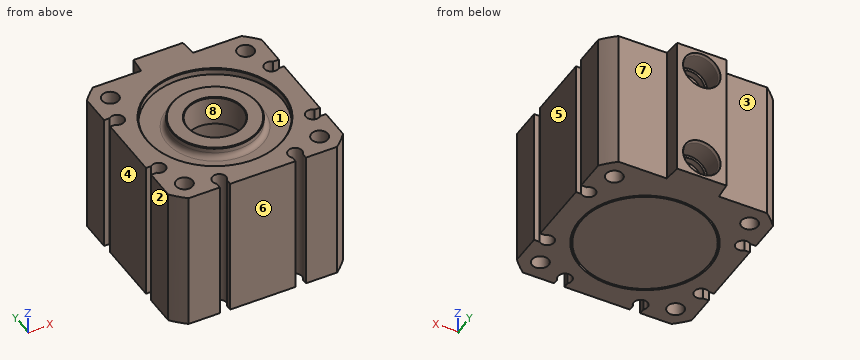
from build123d import *

# Parameters (mm, degrees)
EXTRUDE1_DEPTH                               = 20.701
EXTRUDE1_DEPTH_BACK                          = 20.701
SKETCH1_W                                    = 50.8
SKETCH1_H                                    = 50.8
F_056_250_NOSE_CHAMFER_R                     = 1.5
SKETCH13_R                                   = 35.921024484
SKETCH13_R_2                                 = 33.34
F_075_250_TUBE_EDGE_ROUNDOVER_DEPTH          = 55.812823354
F_075_250_PORT_BOSS_DEPTH                    = 41.402
F_106_200_PORT_1_8_NPT_AT_2_COUNT            = 2
F_106_200_PORT_1_8_NPT_AT_2_PITCH            = 28.702
F_075_250_SWITCH_GROOVE_DEPTH                = 58.174392905
F_075_106_SWITCH_GROOVE_CIRC_PATTERN_COUNT   = 3
F_075_106_SWITCH_GROOVE_CIRC_PATTERN_ANGLE   = 180
SKETCH19_W                                   = 0.15
SKETCH19_H                                   = 19
F_075_250_THIN_SIDE_CUTS_DEPTH               = 58.174392905
SKETCH20_R                                   = 1.9
F_075_250_MOUNT_THRU_HOLE_DEPTH              = 58.174392905
F_075_250_MOUNT_THRU_HOLE_CIRC_PATTERN_COUNT = 4
F_150_10_24_A_MOUNT_TAPPED_AT_2_COUNT        = 2
F_150_10_24_A_MOUNT_TAPPED_AT_2_PITCH        = 39.29
F_150_10_24_A_MOUNT_TAPPED_AT_3_COUNT        = 2
F_150_10_24_A_MOUNT_TAPPED_AT_3_PITCH        = 55.564450866
F_150_10_24_A_MOUNT_TAPPED_AT_4_COUNT        = 2
F_150_10_24_A_MOUNT_TAPPED_AT_4_PITCH        = 39.29
F_056_250_START                              = -12.025
SKETCH22_R                                   = 19.05
F_056_250_STROKE_CHAMBER_DEPTH               = 24.05
SKETCH23_R                                   = 8.001
F_056_250_ROD_THRU_BORE_DEPTH                = 45.534447353
SKETCH41_R                                   = 19.05
SKETCH41_R_2                                 = 18.55
END_PLATE_DEPTH                              = 1
END_PLATE_TAPER                              = 30
F_056_250_COLLAR_CHAMFER_SIZE                = 0.2


with BuildPart() as part:
    # Sketch1 → Extrude1 (new, two sides: drawn at the far end of the back side and taken through both)
    with BuildSketch(Plane.XY.offset(-EXTRUDE1_DEPTH_BACK)):
        Rectangle(SKETCH1_W, SKETCH1_H)
    extrude(amount=EXTRUDE1_DEPTH + EXTRUDE1_DEPTH_BACK)

    # Sketch33 → 056-250 Front Recess (revolve, cut)
    with BuildSketch(Plane(origin=(0, 0, 0), x_dir=(0, 0, -1), z_dir=(1, 0, 0)), mode=Mode.PRIVATE) as f_056_250_front_recess_sk:
        Polygon((-20.701, 19.55), (-18.801, 19.55), (-18.801, 21), (-17.651, 21), (-17.651, 12.5), (-20.701, 12.5), align=None)
    revolve(f_056_250_front_recess_sk.sketch.rotate(Axis((0, 0, 61.220394237), (0, 0, -1)), 90), axis=Axis((0, 0, 61.220394237), (0, 0, -1)), mode=Mode.SUBTRACT)

    # 056-250 Nose Chamfer
    f_056_250_nose_chamfer_edges = [part.edges().sort_by_distance(p)[0] for p in [
        (-12.5, 0, 17.651),
    ]]
    fillet(f_056_250_nose_chamfer_edges, radius=F_056_250_NOSE_CHAMFER_R)

    # Sketch13 → 075-250 Tube Edge Roundover (cut, through all)
    with BuildSketch(Plane.XY.offset(20.701)):
        Circle(SKETCH13_R)
        Circle(SKETCH13_R_2, mode=Mode.SUBTRACT)
    extrude(amount=-F_075_250_TUBE_EDGE_ROUNDOVER_DEPTH, mode=Mode.SUBTRACT)

    # Sketch14 → 075-250 Port Boss (add)
    with BuildSketch(Plane.XY.offset(20.701)):
        Polygon((-7.15, 30.16), (7.15, 30.16), (7.566446038, 25.4), (-7.566446038, 25.4), align=None)
    extrude(amount=-F_075_250_PORT_BOSS_DEPTH)

    # Sketch36 → 106-200 Port 1/8 NPT (revolve, cut)
    with BuildSketch(Plane(origin=(0, 30.16, 14.351), x_dir=(0, 0, 1), z_dir=(1, 0, 0))):
        Polygon((0, 0), (0, 10.533468714), (4.2164, 8), (4.2164, 6.2), (4.959907269, 6.2), (5.1218211, 0.792298297), (5.4500018, 0), align=None)
    f_106_200_port_1_8_npt = revolve(axis=Axis((0, 36.51, 14.351), (0, -1, 0)), mode=Mode.SUBTRACT)

    # 106-200 Port 1/8 NPT at 2: 106-200 Port 1/8 NPT ×2
    with Locations(*[(0, 0, -i * F_106_200_PORT_1_8_NPT_AT_2_PITCH) for i in range(1, F_106_200_PORT_1_8_NPT_AT_2_COUNT)]):
        add(f_106_200_port_1_8_npt, mode=Mode.SUBTRACT)

    # Sketch15 → 075-250 Switch Groove (cut, through all)
    with BuildSketch(Plane.XY.offset(20.701)):
        with BuildLine():
            Line((-25.4, 12.5), (-23.760376786, 12.5))
            ThreePointArc((-23.760376786, 12.5), (-20.375, 11), (-23.760376786, 9.5))
            Line((-23.760376786, 9.5), (-25.4, 9.5))
            Line((-25.4, 9.5), (-25.4, 12.5))
        make_face()
        with BuildLine():
            Line((-25.4, -12.5), (-25.4, -9.5))
            Line((-25.4, -9.5), (-23.760376786, -9.5))
            ThreePointArc((-23.760376786, -9.5), (-20.375, -11), (-23.760376786, -12.5))
            Line((-23.760376786, -12.5), (-25.4, -12.5))
        make_face()
    f_075_250_switch_groove = extrude(amount=-F_075_250_SWITCH_GROOVE_DEPTH, mode=Mode.SUBTRACT)

    # 075-106 Switch Groove Circ Pattern: 075-250 Switch Groove ×3 about axis
    f_075_106_switch_groove_circ_pattern_axis = Axis((0, 0, 0), (0, 0, 1))
    for i in range(1, F_075_106_SWITCH_GROOVE_CIRC_PATTERN_COUNT):
        add(f_075_250_switch_groove.rotate(f_075_106_switch_groove_circ_pattern_axis, i * F_075_106_SWITCH_GROOVE_CIRC_PATTERN_ANGLE / (F_075_106_SWITCH_GROOVE_CIRC_PATTERN_COUNT - 1)), mode=Mode.SUBTRACT)

    # Sketch19 → 075-250 Thin Side Cuts (cut, through all)
    with BuildSketch(Plane.XY.offset(20.701)):
        with Locations((25.325, 0)):
            Rectangle(SKETCH19_W, SKETCH19_H)
        with Locations((-25.325, 0)):
            Rectangle(SKETCH19_W, SKETCH19_H)
    extrude(amount=-F_075_250_THIN_SIDE_CUTS_DEPTH, mode=Mode.SUBTRACT)

    # Sketch20 → 075-250 Mount Thru Hole (cut, through all)
    with BuildSketch(Plane.XY.offset(20.701)):
        with Locations((19.645, 19.645)):
            Circle(SKETCH20_R)
    f_075_250_mount_thru_hole = extrude(amount=-F_075_250_MOUNT_THRU_HOLE_DEPTH, mode=Mode.SUBTRACT)

    # 075-250 Mount Thru Hole Circ Pattern: 075-250 Mount Thru Hole ×4 about axis
    f_075_250_mount_thru_hole_circ_pattern_axis = Axis((0, 0, 0), (0, 0, 1))
    for i in range(1, F_075_250_MOUNT_THRU_HOLE_CIRC_PATTERN_COUNT):
        add(f_075_250_mount_thru_hole.rotate(f_075_250_mount_thru_hole_circ_pattern_axis, i * 360 / F_075_250_MOUNT_THRU_HOLE_CIRC_PATTERN_COUNT), mode=Mode.SUBTRACT)

    # Sketch28 → 150 #10-24 A Mount Tapped (revolve, cut)
    with BuildSketch(Plane(origin=(19.645, 19.645, 20.701), x_dir=(0, -1, 0), z_dir=(1, 0, 0))):
        Polygon((0, 0), (0, 17.018324014), (1.89865, 15.8775), (1.89865, 12.7), (2.413, 12.7), (2.413, 0), align=None)
    f_150_10_24_a_mount_tapped = revolve(axis=Axis((19.645, 19.645, 27.051), (0, 0, -1)), mode=Mode.SUBTRACT)

    # 150 #10-24 A Mount Tapped at 2: 150 #10-24 A Mount Tapped ×2
    with Locations(*[(-i * F_150_10_24_A_MOUNT_TAPPED_AT_2_PITCH, 0, 0) for i in range(1, F_150_10_24_A_MOUNT_TAPPED_AT_2_COUNT)]):
        add(f_150_10_24_a_mount_tapped, mode=Mode.SUBTRACT)

    # 150 #10-24 A Mount Tapped at 3: 150 #10-24 A Mount Tapped ×2
    with Locations(*[Vector(-0.7071067811865451, -0.7071067811865499, 0) * (i * F_150_10_24_A_MOUNT_TAPPED_AT_3_PITCH) for i in range(1, F_150_10_24_A_MOUNT_TAPPED_AT_3_COUNT)]):
        add(f_150_10_24_a_mount_tapped, mode=Mode.SUBTRACT)

    # 150 #10-24 A Mount Tapped at 4: 150 #10-24 A Mount Tapped ×2
    with Locations(*[(0, -i * F_150_10_24_A_MOUNT_TAPPED_AT_4_PITCH, 0) for i in range(1, F_150_10_24_A_MOUNT_TAPPED_AT_4_COUNT)]):
        add(f_150_10_24_a_mount_tapped, mode=Mode.SUBTRACT)

    # 150 #10-24 A Mount Tapped to Rear: 150 #10-24 A Mount Tapped across plane
    add(f_150_10_24_a_mount_tapped.mirror(Plane.XY), mode=Mode.SUBTRACT)

    # 150 #10-24 A Mount Tapped to Rear copy 1 → 150 #10-24 A Mount Tapped to Rear co 2 (revolve, cut)
    with BuildSketch(Plane(origin=(-19.645, 19.645, -20.701), x_dir=(0, -1, 0), z_dir=(1, 0, 0))):
        Polygon((0, 0), (0, -17.018324014), (1.89865, -15.8775), (1.89865, -12.7), (2.413, -12.7), (2.413, 0), align=None)
    revolve(axis=Axis((-19.645, 19.645, -27.051), (0, 0, -1)), mode=Mode.SUBTRACT)

    # 150 #10-24 A Mount Tapped to Rear copy 2 → 150 #10-24 A Mount Tapped to Rear co 3 (revolve, cut)
    with BuildSketch(Plane(origin=(-19.645, -19.645, -20.701), x_dir=(0, -1, 0), z_dir=(1, 0, 0))):
        Polygon((0, 0), (0, -17.018324014), (1.89865, -15.8775), (1.89865, -12.7), (2.413, -12.7), (2.413, 0), align=None)
    revolve(axis=Axis((-19.645, -19.645, -27.051), (0, 0, -1)), mode=Mode.SUBTRACT)

    # 150 #10-24 A Mount Tapped to Rear copy 3 → 150 #10-24 A Mount Tapped to Rear co 4 (revolve, cut)
    with BuildSketch(Plane(origin=(19.645, -19.645, -20.701), x_dir=(0, -1, 0), z_dir=(1, 0, 0))):
        Polygon((0, 0), (0, -17.018324014), (1.89865, -15.8775), (1.89865, -12.7), (2.413, -12.7), (2.413, 0), align=None)
    revolve(axis=Axis((19.645, -19.645, -27.051), (0, 0, -1)), mode=Mode.SUBTRACT)

    # Sketch22 → 056-250 Stroke Chamber (cut)
    with BuildSketch(Plane.XY.offset(F_056_250_START)):
        Circle(SKETCH22_R)
    extrude(amount=F_056_250_STROKE_CHAMBER_DEPTH, mode=Mode.SUBTRACT)

    # Sketch23 → 056-250 Rod Thru Bore (cut, through all)
    with BuildSketch(Plane.XY):
        Circle(SKETCH23_R)
    extrude(amount=F_056_250_ROD_THRU_BORE_DEPTH, mode=Mode.SUBTRACT)

    # Sketch41 → End Plate (cut)
    with BuildSketch(Plane(origin=(0, 0, -20.701), x_dir=(-1, 0, 0), z_dir=(0, 0, -1))):
        with Locations(Location((0, 0, 0), (0, 0, 180))):
            Circle(SKETCH41_R)
        Circle(SKETCH41_R_2, mode=Mode.SUBTRACT)
    extrude(amount=-END_PLATE_DEPTH, taper=END_PLATE_TAPER, mode=Mode.SUBTRACT)

    # 056-250 Collar Chamfer
    f_056_250_collar_chamfer_edges = [part.edges().sort_by_distance(p)[0] for p in [
        (-19.55, 0, 20.701),
        (-12.5, 0, 20.701),
        (-8.001, 0, 20.701),
    ]]
    chamfer(f_056_250_collar_chamfer_edges, length=F_056_250_COLLAR_CHAMFER_SIZE)


solid = part.part
Here's how the part is built. I have some questions about the finished solid (model axes, mm). Face numbers are marked on the shaded views. A direction names the side the tool comes from. Round coordinates to 2 decimals unless told otherwise and drop trailing zeros.
1. Suppose I cut it at A-A (z = -1.5). State how many separate pieces and enclosed holes the cut face has, and give its area (3 significant figures).
2. Will these pins go through, and if not, where does the flat tip stop? pin 1 Ø1.8 at (x, z) = (-24.5, -8) entering from +Y; pin 2 Ø1.8 at (x, z) = (-24.5, -3.5) entering from -Y; pin 3 Ø15 at (y, z) = (-0.5, 5.5) entering from -X.
3. I need wall thicknesses on L1, parallel to X at y = -19.5, z = 10; L2, parallel to X at y = 20, z = -6.5; L3, parallel to Y at x = 22.5, z = -12. Which ranges of each line are inside material? Lowest first, please.
4. If we mould it in two halves opening along Y, with no side actions, what happens to the marked faces 5, 6, 7 and 8? For each: released by +Y, released by -Y, zero draft, split by the parting line, or undercut.
5. For the marked faces 1, 2, 3 and 4, which set-ups out of +Z, -Z, +X, -X, +Y, -Y let a thin tool reach every point of the face, with its end or its side?
Answer sheet:
1. separate pieces: 1
1. enclosed holes: 5
1. area: 1,330 mm2
2. pin 1: stops at y = 23.55
2. pin 2: stops at y = -23.55
2. pin 3: stops at x = -25.25
3. L1: x = -25.4 to -22.05, -17.24 to 17.24, 22.05 to 25.4
3. L2: x = -25.4 to -21.51, -17.78 to 17.78, 21.51 to 25.4
3. L3: y = -24.6 to -13.02, -8.98 to 8.98, 13.02 to 24.6
4. face 5: undercut
4. face 6: released by -Y
4. face 7: released by +Y
4. face 8: undercut
5. face 1: none
5. face 2: +Z, -Z, -X, +Y, -Y
5. face 3: +Z, -Z, -X, +Y
5. face 4: +Z, -Z, -X
